CAD build for the part. Positions are in the model's coordinates, mm. Face numbers are marked on the shaded views. Coordinates: 2 decimals unless noted, no trailing zeros. Write each loop counter-clockwise with the first axis right and the second up, starting at its lowest first coordinate (ties: lowest second). Pieces come first, ordered by that corner, then holes. Notation, with made-up numbers: (86, 35.25) -> (97, 35.25) arc R22 ccw to (97, 44.25) -> close; hole circle Ø9 at (13.5, -0.75). An arc over 180 degrees is marked (long way). Answer as CSV lines item,"result".
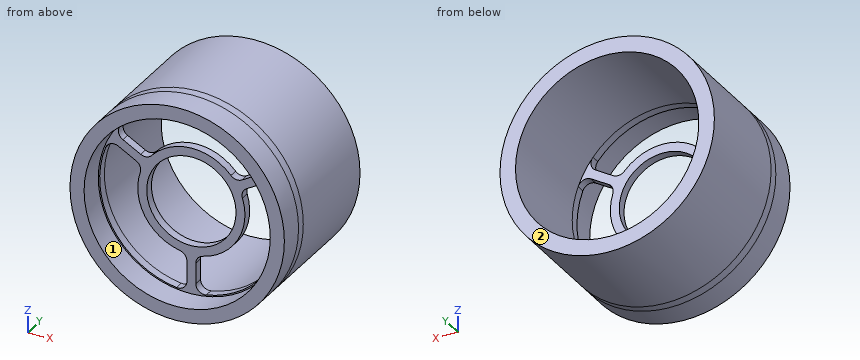
```python
from build123d import *

# Parameters (mm, degrees)
SKETCH1_R           = 38.1
SKETCH1_R_2         = 33.0835
BOSS_EXTRUDE1_DEPTH = 9.525
SKETCH2_R           = 38.1
SKETCH2_R_2         = 15.875
BOSS_EXTRUDE2_DEPTH = 3.175
SKETCH4_R           = 38.1
SKETCH4_R_2         = 32.5882
BOSS_EXTRUDE3_DEPTH = 38.1


with BuildPart() as part:
    # Sketch1 → Boss-Extrude1 (new body)
    with BuildSketch(Plane(origin=(0, 0, 0), x_dir=(1, 0, 0), z_dir=(0, 1, 0))):
        Circle(SKETCH1_R)
        Circle(SKETCH1_R_2, mode=Mode.SUBTRACT)
    extrude(amount=-BOSS_EXTRUDE1_DEPTH)

    # Sketch2 → Boss-Extrude2 (add)
    with BuildSketch(Plane(origin=(0, 0, 0), x_dir=(1, 0, 0), z_dir=(0, 1, 0))):
        Circle(SKETCH2_R)
        Circle(SKETCH2_R_2, mode=Mode.SUBTRACT)
        with BuildLine():
            Line((-1.5875, 29.025074125), (-1.5875, 21.708736001))
            ThreePointArc((-1.5875, 21.708736001), (-2.288559931, 19.718699434), (-4.082142857, 18.607488001))
            ThreePointArc((-4.082142857, 18.607488001), (-16.497783942, 9.525), (-18.155628738, -5.768504584))
            ThreePointArc((-18.155628738, -5.768504584), (-18.221174605, -7.877398679), (-19.594066861, -9.479552672))
            Line((-19.594066861, -9.479552672), (-25.930201539, -13.137721734))
            ThreePointArc((-25.930201539, -13.137721734), (-28.585844638, -13.378023404), (-30.488092465, -11.509430788))
            ThreePointArc((-30.488092465, -11.509430788), (-28.222209064, 16.2941), (-5.276586788, 32.158177982))
            ThreePointArc((-5.276586788, 32.158177982), (-2.707214199, 31.445079348), (-1.5875, 29.025074125))
        make_face(mode=Mode.SUBTRACT)
        with BuildLine():
            Line((1.5875, 29.025074125), (1.5875, 21.708736001))
            ThreePointArc((1.5875, 21.708736001), (2.288559931, 19.718699434), (4.082142857, 18.607488001))
            ThreePointArc((4.082142857, 18.607488001), (16.497783942, 9.525), (18.155628738, -5.768504584))
            ThreePointArc((18.155628738, -5.768504584), (18.221174605, -7.877398679), (19.594066861, -9.479552672))
            Line((19.594066861, -9.479552672), (25.930201539, -13.137721734))
            ThreePointArc((25.930201539, -13.137721734), (28.585844638, -13.378023404), (30.488092465, -11.509430788))
            ThreePointArc((30.488092465, -11.509430788), (28.222209064, 16.2941), (5.276586788, 32.158177982))
            ThreePointArc((5.276586788, 32.158177982), (2.707214199, 31.445079348), (1.5875, 29.025074125))
        make_face(mode=Mode.SUBTRACT)
        with BuildLine():
            Line((24.342701539, -15.887352391), (18.006566861, -12.229183329))
            ThreePointArc((18.006566861, -12.229183329), (15.932614674, -11.841300756), (14.073485881, -12.838983416))
            ThreePointArc((14.073485881, -12.838983416), (0, -19.05), (-14.073485881, -12.838983416))
            ThreePointArc((-14.073485881, -12.838983416), (-15.932614674, -11.841300756), (-18.006566861, -12.229183329))
            Line((-18.006566861, -12.229183329), (-24.342701539, -15.887352391))
            ThreePointArc((-24.342701539, -15.887352391), (-25.87863044, -18.067055943), (-25.211505678, -20.648747194))
            ThreePointArc((-25.211505678, -20.648747194), (0, -32.5882), (25.211505678, -20.648747194))
            ThreePointArc((25.211505678, -20.648747194), (25.87863044, -18.067055943), (24.342701539, -15.887352391))
        make_face(mode=Mode.SUBTRACT)
    extrude(amount=BOSS_EXTRUDE2_DEPTH)

    # Sketch4 → Boss-Extrude3 (add)
    with BuildSketch(Plane(origin=(0, 3.175, 0), x_dir=(1, 0, 0), z_dir=(0, 1, 0))):
        Circle(SKETCH4_R)
        Circle(SKETCH4_R_2, mode=Mode.SUBTRACT)
    extrude(amount=BOSS_EXTRUDE3_DEPTH)


solid = part.part
```
Item 1: Flat gauge pins, fed straight in: pin 1 (10 mm diameter, centred on x = -3, z = 20.5, fed in from +Y) (3 decimals); pin 2 (20 mm diameter, centred on x = -11.5, z = 9.5, fed in from -Y); pin 3 (4 mm diameter, centred on x = 6.5, y = 0, fed in from +Z); pin 4 (12 mm diameter, centred on x = 21, z = -24, fed in from -Y) (3 decimals). Where does each tip first touch, or does it go through?
Answer below:
pin 1,"stops at y = 3.175"
pin 2,"stops at y = 0"
pin 3,"stops at z = 37.83"
pin 4,"stops at y = -9.525"
Item 2: Saw through at A-A on x = 0. State how many separate pieces and enclosed holes the cut face has, and give its area (3 significant figures).
Answer below:
separate pieces,"3"
enclosed holes,"0"
area,"614 mm2"
Item 3: Saw through at C-C on x = -9. Give the cut face in (y, z) (3 decimals).
Answer below:
outline,"(-9.525, -37.022) -> (41.275, -37.022) -> (41.275, -31.321) -> (0, -31.321) -> (0, -31.836) -> (-9.525, -31.836) -> close; (-9.525, 31.836) -> (0, 31.836) -> (0, 31.321) -> (41.275, 31.321) -> (41.275, 37.022) -> (-9.525, 37.022) -> close; (0, -16.79) -> (3.175, -16.79) -> (3.175, -13.077) -> (0, -13.077) -> close; (0, 13.077) -> (3.175, 13.077) -> (3.175, 16.79) -> (0, 16.79) -> close"
Item 4: Two-plate mould, pull along Z, no slides. Class the marked faces 1 and 2: pulls with the +Z half, pulls with the -Z half, needs draft (parallel to the pull), parting line crosses it, or undercut.
Answer below:
face 1,"undercut"
face 2,"needs draft"
Item 5: Wall check: line 1 (X direction, y = -7.5, z = 0); line 2 (X direction, y = 1, z = 0) (3 decimals). Give the ranges that are in metal, low to high. Write a range as from..to.
Answer below:
line 1,"x = -38.1..-33.08, 33.08..38.1"
line 2,"x = -38.1..-32.588, -19.05..-15.875, 15.875..19.05, 32.588..38.1"
Item 6: Saw through at D-D on z = 27.5. Give the cut face in (x, y) (3 decimals).
Answer below:
outline,"(-26.37, -9.525) -> (-18.392, -9.525) -> (-18.392, 0) -> (-17.485, 0) -> (-17.485, 41.275) -> (-26.37, 41.275) -> close; (17.485, 0) -> (18.392, 0) -> (18.392, -9.525) -> (26.37, -9.525) -> (26.37, 41.275) -> (17.485, 41.275) -> close"
